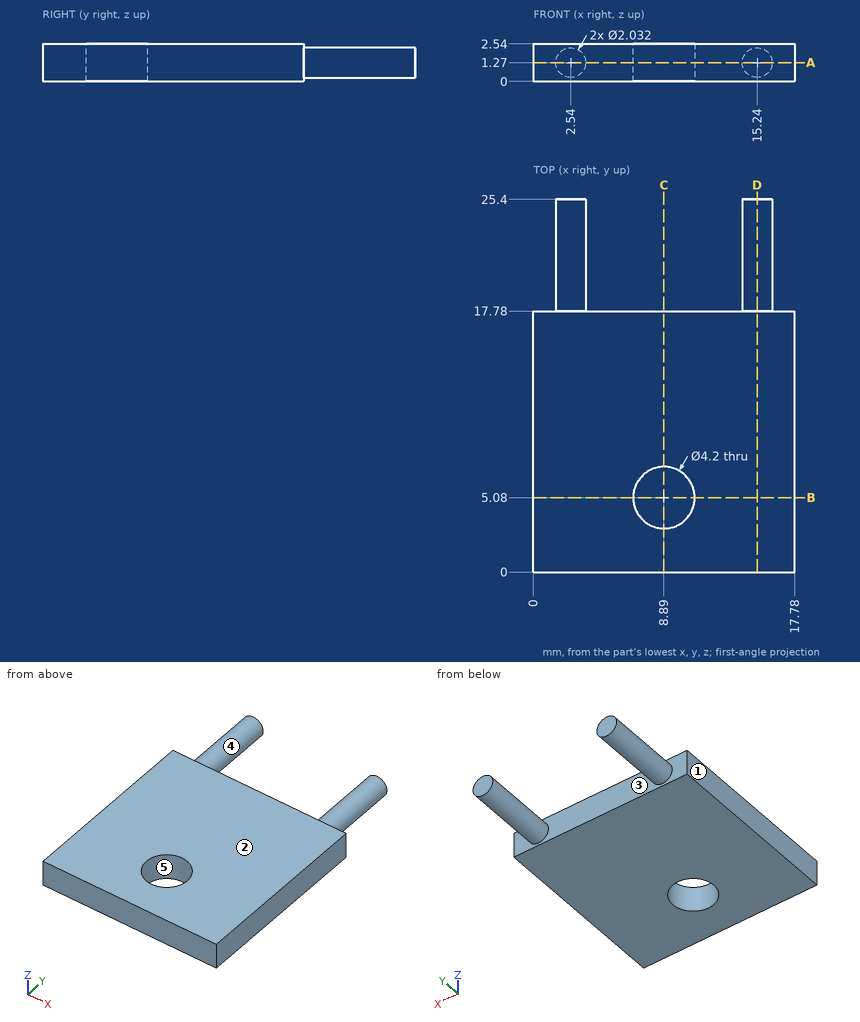
Part print with two shaded views. Sizes in mm from the minimum x, y, z corner. A direction names the side the tool comes from. Give positions to 0.01 mm unless a question says otherwise; leave off trailing zeros. Order: outer loops, then holes, each group sorted by start corner. A loop starts at its lowest first (then second) coordinate and runs counter-clockwise, first axis right, second up.
(1) Saw through at B-B, the plane y = 5.08. Give the cut face in (x, z).
(2) Drill centre lines: L1, parallel to Y at x = 8.89, z = 1.5; L2, parallel to Y at x = 9.5, z = 1.7; L3, parallel to X at y = 3.25, z = 1.7. Where is each one in solid material? Low to high.
(3) Saw through at D-D, the plane x = 15.24. Give the cut face in (y, z), then the cut area to 3 significant figures.
(4) Saw through at A-A, the plane z = 1.27. Give the cut face in (x, y), then the cut area to 3 significant figures.
(5) Mould opens along X. For the marked faces 1, 2 and 3 say: released by +X, released by -X, zero draft, split by the parting line, or undercut.
(6) Tool access for the marked faces 4 and 5: list every direction of +Z, -Z, +X, -X, +Y, -Y with a clear straight run to the whole face (end or side of a thin tool).
(7) Saw through at C-C, the plane x = 8.89. Give the cut face in (y, z), then the cut area to 3 significant figures.
Results found:
1. outline: (0, 0) - (6.79, 0) - (6.79, 2.54) - (0, 2.54) - close; (10.99, 0) - (17.78, 0) - (17.78, 2.54) - (10.99, 2.54) - close
2. L1: y = 0 to 2.98, 7.18 to 17.78
2. L2: y = 0 to 3.07, 7.09 to 17.78
2. L3: x = 0 to 7.86, 9.92 to 17.78
3. outline: (0, 0) - (17.78, 0) - (17.78, 0.25) - (25.4, 0.25) - (25.4, 2.29) - (17.78, 2.29) - (17.78, 2.54) - (0, 2.54) - close
3. area: 60.6 mm2
4. outline: (0, 0) - (17.78, 0) - (17.78, 17.78) - (16.26, 17.78) - (16.26, 25.4) - (14.22, 25.4) - (14.22, 17.78) - (3.56, 17.78) - (3.56, 25.4) - (1.52, 25.4) - (1.52, 17.78) - (0, 17.78) - close; hole circle Ø4.2 at (8.89, 5.08)
4. area: 333 mm2
5. face 1: released by -X
5. face 2: zero draft
5. face 3: undercut
6. face 4: +Y
6. face 5: +Z, -Z
7. outline: (0, 0) - (2.98, 0) - (2.98, 2.54) - (0, 2.54) - close; (7.18, 0) - (17.78, 0) - (17.78, 2.54) - (7.18, 2.54) - close
7. area: 34.5 mm2
